Study the drawing (mm; zero at the part's minimum x, y, z) and answer. A direction names the side the tool comes from. Coordinates: 2 decimals unless noted, no trailing zeros. Order: outer loops, then holes, each group sorted by start corner. A loop starts at its lowest first (then second) coordinate and runs counter-clockwise, first axis right, second up. Notation, with made-up numbers: M 5.25,20.5 L 46.25,20.5 A28 cw 46.25,54.5 Z; hole C -25,82 d7. An arc over 180 degrees is marked long. Use a Markdown table: item, result. Add a question column.
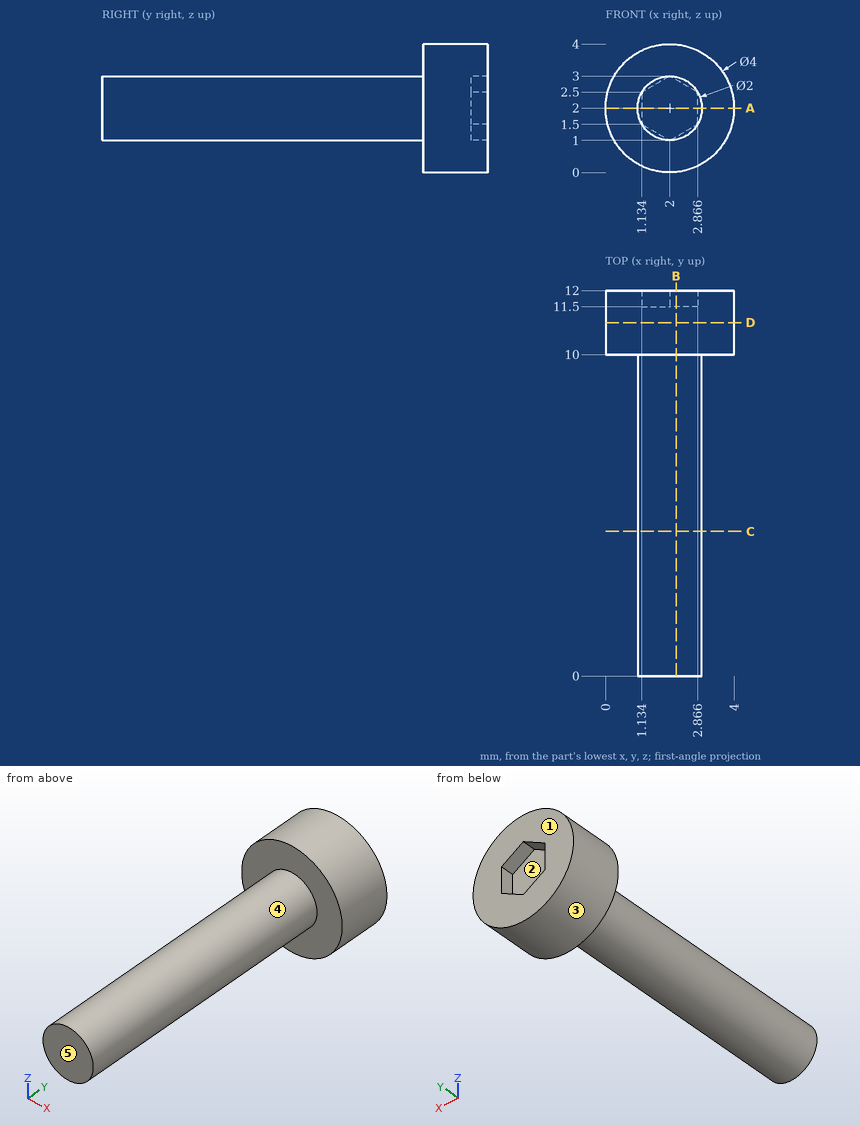
(1) A cutting plane is placed at D-D on y = 11. Write down the section's boundary in (x, z).
(2) Which of the six approach directions +Z, -Z, +X, -X, +Y, -Y give full straight-line access (tool end or side, diameter ignored) to the marked faces 4 and 5?
(3) Straight lines are drawn through the part: line 1 (Y direction, x = 1.35, z = 0.4); line 2 (Z direction, x = 1.5, y = 5.75); line 3 (Z direction, x = 2.65, y = 9.75). For each, find the intervals that lie inside material, in ascending order.
(4) The mould has two halves that part along X. Classify the marked faces 1, 2 and 3: pulls with the +X half, pulls with the -X half, needs draft (parallel to the pull), parting line crosses it, or undercut.
(5) A cutting plane is placed at C-C on y = 4.5. Write down the section's boundary in (x, z).
(6) Given P1, Ø1, axis at x = 1, y = 5, coming from the -Z side, flat-ended and moving along its own axis, determine where the tip first touches the part or whether it passes through.
(7) A cutting plane is placed at A-A on z = 2. Write down the section's boundary in (x, y), plus the area to 3 significant figures.
(8) A cutting plane is placed at B-B on x = 2.2. Write down the section's boundary in (y, z), plus the area to 3 significant figures.
From the geometry:
| question | item | result |
|---|---|---|
| 1 | outline | C 2,2 d4 |
| 2 | face 4 | -Y |
| 2 | face 5 | +Z, -Z, +X, -X, -Y |
| 3 | line 1 | y = 10 to 12 |
| 3 | line 2 | z = 1.13 to 2.87 |
| 3 | line 3 | z = 1.24 to 2.76 |
| 4 | face 1 | needs draft |
| 4 | face 2 | undercut |
| 4 | face 3 | parting line crosses it |
| 5 | outline | C 2,2 d2 |
| 6 | P1 | stops at z = 1.13 |
| 7 | outline | M 0,10 L 1,10 L 1,0 L 3,0 L 3,10 L 4,10 L 4,12 L 2.87,12 L 2.87,11.5 L 1.13,11.5 L 1.13,12 L 0,12 Z |
| 7 | area | 27.1 mm2 |
| 8 | outline | M 0,1.02 L 10,1.02 L 10,0.01 L 12,0.01 L 12,1.12 L 11.5,1.12 L 11.5,2.88 L 12,2.88 L 12,3.99 L 10,3.99 L 10,2.98 L 0,2.98 Z |
| 8 | area | 26.7 mm2 |
